Check sheet for the modelled part. Datum: model origin and axes. Units: mm. A direction names the side the tool comes from. Give positions to 0.01 mm unless a question says otherwise; leave off trailing zeros. Write each loop counter-clockwise with the first axis right and the second up, starting at its lowest first coordinate (ties: lowest second). Pieces come first, ordered by that corner, then holes. Notation, with made-up numbers: M 58,9 L 97,9 A21 cw 97,22 Z; hole C 51,44.5 d2. An arc over 180 degrees is marked long. Write each question's results on one line, items separated by ' | '. Start each with the question number.
from build123d import *
from OCP.BRepFilletAPI import BRepFilletAPI_MakeChamfer

# Parameters (mm, degrees)
SKIZZE1_R                          = 1.65
SKIZZE1_R_2                        = 2.25
AUFSATZ_LINEAR_AUSTRAGEN1_DEPTH    = 3
SKIZZE2_W                          = 128
SKIZZE2_H                          = 2
SKIZZE2_R                          = 2.25
AUFSATZ_LINEAR_AUSTRAGEN2_DEPTH    = 10
FASE1_SIZE                         = 1.732050808
FASE1_SIZE_2                       = 3
FASE2_SIZE                         = 1.732050808
FASE2_SIZE_2                       = 3
SCHNITT_LINEAR_START               = -5
SCHNITT_LINEAR_AUSTRAGEN1_DEPTH    = 3
SCHNITT_LINEAR_START_2             = -41.26795
SCHNITT_LINEAR_AUSTRAGEN2_DEPTH    = 3
SCHNITT_LINEAR_START_3             = -8
SCHNITT_LINEAR_AUSTRAGEN3_DEPTH    = 3
SCHNITT_LINEAR_START_4             = -44.26795
SCHNITT_LINEAR_AUSTRAGEN4_DEPTH    = 3
K_RPER_VERSCHIEBEN_KOPIEREN1_ANGLE = 90


# Some blends are built 0.0001 mm under size
with BuildPart() as part:
    # Skizze1 → Aufsatz-Linear austragen1 (new body)
    with BuildSketch(Plane(origin=(0, 0, 0), x_dir=(1, 0, 0), z_dir=(0, 1, 0))):
        Polygon((54, -20), (74, -20), (74, -30), (128, -30), (128, 0), (0, 0), (0, -30), (54, -30), align=None)
        with Locations(Location((114, -10, 0), (0, 0, 90))):
            Circle(SKIZZE1_R, mode=Mode.SUBTRACT)
        with Locations(Location((14, -10, 0), (0, 0, 270))):
            Circle(SKIZZE1_R, mode=Mode.SUBTRACT)
        with Locations(Location((29, -13, 0), (0, 0, 270))):
            Circle(SKIZZE1_R_2, mode=Mode.SUBTRACT)
        with Locations(Location((99, -13, 0), (0, 0, 270))):
            Circle(SKIZZE1_R_2, mode=Mode.SUBTRACT)
    extrude(amount=AUFSATZ_LINEAR_AUSTRAGEN1_DEPTH)

    # Skizze2 → Aufsatz-Linear austragen2 (add)
    # profile 1 of 3: a face of its own
    with BuildSketch(Plane(origin=(0, 3, 0), x_dir=(1, 0, 0), z_dir=(0, 1, 0))):
        with Locations((64, -1)):
            Rectangle(SKIZZE2_W, SKIZZE2_H)
    # profile 2 of 3: a face of its own
    with BuildSketch(Plane(origin=(0, 3, 0), x_dir=(1, 0, 0), z_dir=(0, 1, 0))):
        with BuildLine():
            Line((0, -9.5), (10.031373033, -9.5))
            ThreePointArc((10.031373033, -9.5), (14, -14), (17.968626967, -9.5))
            Line((17.968626967, -9.5), (54, -9.5))
            Line((54, -9.5), (54, -18))
            Line((54, -18), (0, -18))
            Line((0, -18), (0, -9.5))
        make_face()
        with Locations(Location((29, -13, 0), (0, 0, 270))):
            Circle(SKIZZE2_R, mode=Mode.SUBTRACT)
    # profile 3 of 3: a face of its own
    with BuildSketch(Plane(origin=(0, 3, 0), x_dir=(1, 0, 0), z_dir=(0, 1, 0))):
        with BuildLine():
            Line((128, -9.5), (128, -18))
            Line((128, -18), (74, -18))
            Line((74, -18), (74, -9.5))
            Line((74, -9.5), (110.031373033, -9.5))
            ThreePointArc((110.031373033, -9.5), (114, -14), (117.968626967, -9.5))
            Line((117.968626967, -9.5), (128, -9.5))
        make_face()
        with Locations(Location((99, -13, 0), (0, 0, 270))):
            Circle(SKIZZE2_R, mode=Mode.SUBTRACT)
    extrude(amount=AUFSATZ_LINEAR_AUSTRAGEN2_DEPTH)

    # Fase1
    fase1_edges_1 = [part.edges().sort_by_distance(p)[0] for p in [
        (54, 8, 9.5),
    ]]
    fase1_side_1 = [part.faces().sort_by_distance(p)[0] for p in [
        (53.965358984, 8, 9.5),
    ]]
    fase1_edges_2 = [part.edges().sort_by_distance(p)[0] for p in [
        (74, 8, 9.5),
    ]]
    fase1_side_2 = [part.faces().sort_by_distance(p)[0] for p in [
        (74, 8, 9.534641016),
    ]]
    fase1_edges_3 = [part.edges().sort_by_distance(p)[0] for p in [
        (64, 3, 2),
    ]]
    fase1_side_3 = [part.faces().sort_by_distance(p)[0] for p in [
        (64, 3, 2.034641016),
    ]]
    fase1_edges_4 = [part.edges().sort_by_distance(p)[0] for p in [
        (27, 3, 18),
    ]]
    fase1_side_4 = [part.faces().sort_by_distance(p)[0] for p in [
        (27, 3, 18.034641016),
    ]]
    fase1_edges_5 = [part.edges().sort_by_distance(p)[0] for p in [
        (101, 3, 18),
    ]]
    fase1_side_5 = [part.faces().sort_by_distance(p)[0] for p in [
        (101, 3, 18.034641016),
    ]]
    fase1_edges_6 = [part.edges().sort_by_distance(p)[0] for p in [
        (27, 3, 30),
    ]]
    fase1_side_6 = [part.faces().sort_by_distance(p)[0] for p in [
        (27, 3, 29.965358984),
    ]]
    fase1_edges_7 = [part.edges().sort_by_distance(p)[0] for p in [
        (101, 3, 30),
    ]]
    fase1_side_7 = [part.faces().sort_by_distance(p)[0] for p in [
        (101, 3, 29.965358984),
    ]]
    fase1 = BRepFilletAPI_MakeChamfer(part.part.solid().wrapped)
    for e in fase1_edges_1:
        fase1.Add(FASE1_SIZE - 0.0001, FASE1_SIZE_2 - 0.0001, e.wrapped, fase1_side_1[0].wrapped)
    for e in fase1_edges_2:
        fase1.Add(FASE1_SIZE_2 - 0.0001, FASE1_SIZE - 0.0001, e.wrapped, fase1_side_2[0].wrapped)
    for e in fase1_edges_3:
        fase1.Add(FASE1_SIZE - 0.0001, FASE1_SIZE_2 - 0.0001, e.wrapped, fase1_side_3[0].wrapped)
    for e in fase1_edges_4:
        fase1.Add(FASE1_SIZE - 0.0001, FASE1_SIZE_2 - 0.0001, e.wrapped, fase1_side_4[0].wrapped)
    for e in fase1_edges_5:
        fase1.Add(FASE1_SIZE - 0.0001, FASE1_SIZE_2 - 0.0001, e.wrapped, fase1_side_5[0].wrapped)
    for e in fase1_edges_6:
        fase1.Add(FASE1_SIZE - 0.0001, FASE1_SIZE_2 - 0.0001, e.wrapped, fase1_side_6[0].wrapped)
    for e in fase1_edges_7:
        fase1.Add(FASE1_SIZE - 0.0001, FASE1_SIZE_2 - 0.0001, e.wrapped, fase1_side_7[0].wrapped)
    add(Compound.cast(fase1.Shape()), mode=Mode.REPLACE)  # a hair under: the kernel refuses the full size

    # Fase2
    # the kernel refuses this chamfer: 3, 1.732050808 mm, written as the material it takes off along each edge
    with BuildSketch(Plane(origin=(54, 3, 20), x_dir=(0, 0.057893862402670915, -0.9983227437537925), z_dir=(1, 0, 0))) as fase2_piece_1:
        Polygon((FASE2_SIZE * 0.998322743505, -FASE2_SIZE * 0.0578938623883), (-FASE2_SIZE_2 * 0.0578938624027, -FASE2_SIZE_2 * 0.998322743754), (0, 0), align=None)
    extrude(amount=20, mode=Mode.SUBTRACT)

    # Skizze3 → Schnitt-Linear austragen1 (cut)
    with BuildSketch(Plane(origin=(128, 0, 0), x_dir=(0, 0, -1), z_dir=(1, 0, 0)).offset(SCHNITT_LINEAR_START)):
        with BuildLine():
            Line((-9.5, 3), (-8.1, 3))
            ThreePointArc((-8.1, 3), (-7.807106781, 2.292893219), (-7.1, 2))
            Line((-7.1, 2), (-6.132050808, 2))
            ThreePointArc((-6.132050808, 2), (-5.424944026, 2.292893219), (-5.132050808, 3))
            Line((-5.132050808, 3), (-3.732050808, 3))
            ThreePointArc((-3.732050808, 3), (-4.434994533, 1.302943725), (-6.132050808, 0.6))
            Line((-6.132050808, 0.6), (-7.1, 0.6))
            ThreePointArc((-7.1, 0.6), (-8.797056275, 1.302943725), (-9.5, 3))
        make_face()
    extrude(amount=-SCHNITT_LINEAR_AUSTRAGEN1_DEPTH, mode=Mode.SUBTRACT)

    # Skizze4 → Schnitt-Linear austragen2 (cut)
    with BuildSketch(Plane(origin=(120, 0, 0), x_dir=(0, 0, -1), z_dir=(1, 0, 0)).offset(SCHNITT_LINEAR_START_2)):
        with BuildLine():
            Line((-7.1, 0.6), (-6.132050808, 0.6))
            ThreePointArc((-6.132050808, 0.6), (-4.434994533, 1.302943725), (-3.732050808, 3))
            Line((-3.732050808, 3), (-5.132050808, 3))
            ThreePointArc((-5.132050808, 3), (-5.424944026, 2.292893219), (-6.132050808, 2))
            Line((-6.132050808, 2), (-7.1, 2))
            ThreePointArc((-7.1, 2), (-7.807106781, 2.292893219), (-8.1, 3))
            Line((-8.1, 3), (-9.5, 3))
            ThreePointArc((-9.5, 3), (-8.797056275, 1.302943725), (-7.1, 0.6))
        make_face()
    extrude(amount=-SCHNITT_LINEAR_AUSTRAGEN2_DEPTH, mode=Mode.SUBTRACT)

    # Skizze5 → Schnitt-Linear austragen3 (cut)
    with BuildSketch(Plane.ZY.offset(SCHNITT_LINEAR_START_3)):
        with BuildLine():
            Line((9.5, 3), (8.1, 3))
            ThreePointArc((8.1, 3), (7.807106781, 2.292893219), (7.1, 2))
            Line((7.1, 2), (6.132050808, 2))
            ThreePointArc((6.132050808, 2), (5.424944026, 2.292893219), (5.132050808, 3))
            Line((5.132050808, 3), (3.732050808, 3))
            ThreePointArc((3.732050808, 3), (4.434994533, 1.302943725), (6.132050808, 0.6))
            Line((6.132050808, 0.6), (7.1, 0.6))
            ThreePointArc((7.1, 0.6), (8.797056275, 1.302943725), (9.5, 3))
        make_face()
    extrude(amount=SCHNITT_LINEAR_AUSTRAGEN3_DEPTH, mode=Mode.SUBTRACT)

    # Skizze6 → Schnitt-Linear austragen4 (cut)
    with BuildSketch(Plane.ZY.offset(-8).offset(SCHNITT_LINEAR_START_4)):
        with BuildLine():
            Line((9.5, 3), (8.1, 3))
            ThreePointArc((8.1, 3), (7.807106781, 2.292893219), (7.1, 2))
            Line((7.1, 2), (6.132050808, 2))
            ThreePointArc((6.132050808, 2), (5.424944026, 2.292893219), (5.132050808, 3))
            Line((5.132050808, 3), (3.732050808, 3))
            ThreePointArc((3.732050808, 3), (4.434994533, 1.302943725), (6.132050808, 0.6))
            Line((6.132050808, 0.6), (7.1, 0.6))
            ThreePointArc((7.1, 0.6), (8.797056275, 1.302943725), (9.5, 3))
        make_face()
    extrude(amount=SCHNITT_LINEAR_AUSTRAGEN4_DEPTH, mode=Mode.SUBTRACT)


with BuildPart() as part_1:
    # Körper-Verschieben/Kopieren1: moved
    add(part.part.rotate(Axis((0, 6.5, 15), (1, 0, 0)), K_RPER_VERSCHIEBEN_KOPIEREN1_ANGLE))


solid = part_1.part
Q1. Section check C-C on y = -2.5. Record the boundary of the cut face in (x, z).
Q2. Section check D-D on x = 58.5. Record the boundary of the cut face in (y, z), plus the area to 3 significant figures.
Q3. Tool access check on faces 1 (the face through (63.104, 18.646, 13.021)), 2 (the face through (27, -2, 11.5)), 3 (the face through (6.52, 17.08, 9.82)), 4 (the face through (54, 4, 15)). Record the directions out of +Z, -Z, +X, -X, +Y, -Y that give a thin tool (end or side, any length) a straight path to the whole face; none if there is none.
Q4. Release check for a two-part mould opening along X. For faces 5 (the face through (93, 12, 16)), 6 (the face through (13.368, 9.976, 9.979)), 7 (the face through (52.268, 15, 10)) record: pulls with the +X half, pulls with the -X half, needs draft (parallel to the pull), parting line crosses it, or undercut.
Q5. Section check A-A on z = 17. Record the boundary of the cut face in (x, y).
Q6. Depth check by flat-ended pin: pin 1 Ø1.5 at (x, y) = (81, 2.5) entering from +Z; pin 2 Ø5.5 at (x, y) = (14, 11.5) entering from +Z; pin 3 Ø3.5 at (x, z) = (98, 17.5) entering from -Y. Enter the tip coordinate at first touch or a pass-through.
Q7. Scan lines: L1, parallel to X at y = 13.5, z = 10.75; L2, parallel to Y at x = 80.5, z = 14.75; L3, parallel to X at y = 8.5, z = 13.5. Record each from-to range of solid material in increasing order.
Check result:
1) outline: M 0,8.5 L 54,8.5 L 54,11.5 L 0,11.5 Z; M 74,8.5 L 128,8.5 L 128,11.5 L 74,11.5 Z
2) outline: M 1.5,8.5 L 21.5,8.5 L 21.5,21.5 L 19.5,21.5 L 19.5,14.5 L 17.77,11.5 L 3.23,11.5 Z | area: 80.0 mm^2
3) face 1: +Z, +X, -X | face 2: +Z, +X, -X, -Y | face 3: none | face 4: +Z, -Y
4) face 5: needs draft | face 6: undercut | face 7: undercut
5) outline: M 0,3.5 L 54,3.5 L 54,9 L 52.27,12 L 17.97,12 A4 cw long 10.03,12 L 0,12 Z; M 0,19.5 L 128,19.5 L 128,21.5 L 0,21.5 Z; M 74,3.5 L 128,3.5 L 128,12 L 117.97,12 A4 cw long 110.03,12 L 75.73,12 L 74,9 Z; hole C 29,8.5 d4.5; hole C 99,8.5 d4.5
6) pin 1: z = 14.07 | pin 2: z = 11.5 | pin 3: y = 3.5
7) L1: 0 to 5, 8 to 49.27, 52.27 to 75.73, 78.73 to 120, 123 to 128 | L2: 3.5 to 12, 19.5 to 21.5 | L3: 0 to 11.35, 16.65 to 26.75, 31.25 to 54, 74 to 96.75, 101.25 to 111.35, 116.65 to 128
